For this review, use the dimensioned drawing (mm, ordinates from the lowest corner) and the shaded views. A direction names the side the tool comes from. Give positions to 0.01 mm unless a question says otherwise; leave off trailing zeros. Order: outer loops, then holes, each group sorted by start corner. A loop starts at its lowest first (then second) coordinate and runs counter-clockwise, first axis right, second up. Notation, with made-up numbers: (45, 1.25) -> (82, 1.25) arc R25 cw to (82, 38.25) -> close; hole circle Ø2 at (55, -20.75). An arc over 180 degrees is marked (long way). One line per item, written item: value. Start each with the question number.
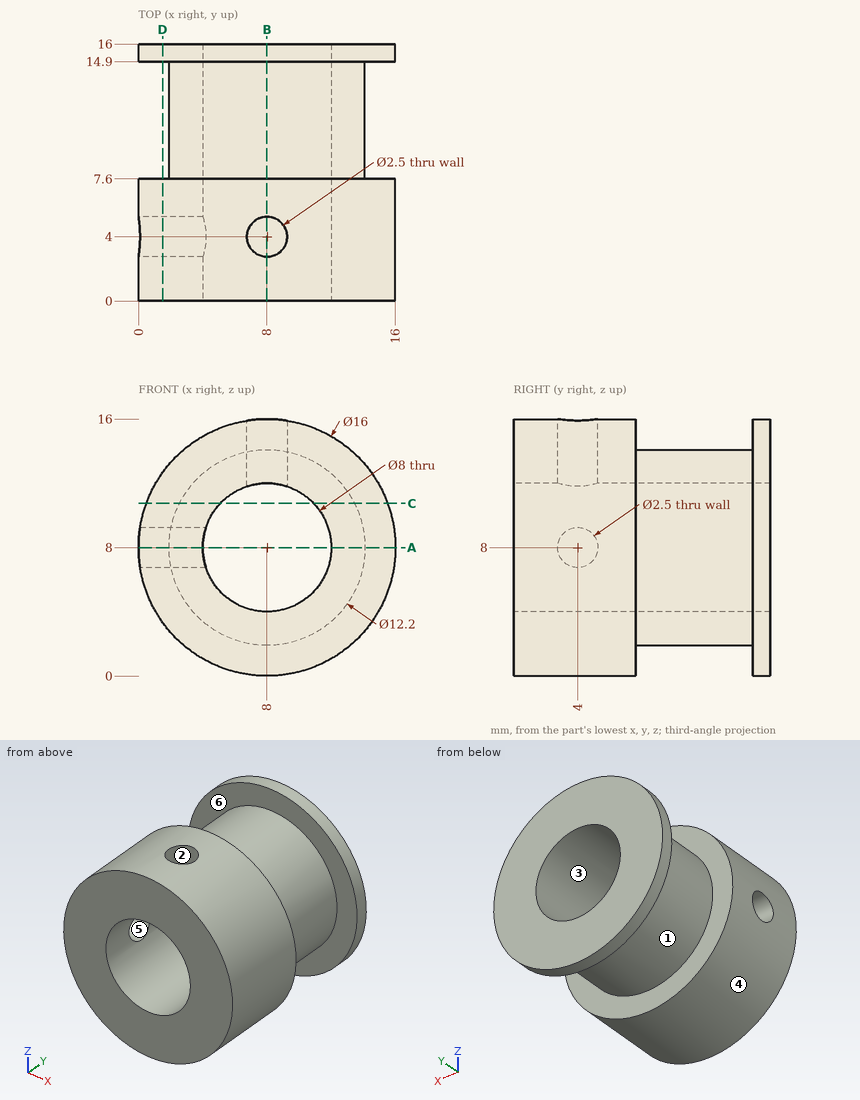
Q1. Take a section at C-C (z = 10.75). State the section outline as (x, y) points.
Q2. Take a section at B-B (x = 8). State the section outline as (y, z) points.
Q3. Take a section at D-D (x = 1.5). State the section outline as (y, z) points, and give its area (3 significant figures).
Q4. Take a section at A-A (z = 8). State the section outline as (x, y) points.
Q5. For the marked faces 4, 5 and 6, list the 3-axis set-ups (+Z, -Z, +X, -X, +Y, -Y) from which the entire face can be reached by the end or side of a thin tool; tool diameter is ignored.
Q6. For line 1 along X through (y, z) = (11.75, 8); line 2 along Y through (x, z) = (4.75, 15); line 3 along Z through (x, y) = (11, 10.5), list the stretches that pass through material, from the lowest coordinate up.
Q7. For pin 1 Ø6 at (y, z) = (7, 6.5) entering from +X; pin 2 Ø3 at (y, z) = (3.5, 10.5) entering from +X; pin 3 Ø4 at (x, y) = (11, 6) entering from -Z; pin 4 Ø3 at (x, y) = (13, 4) entering from +Z, all flat-tipped, find the tip position at first contact; note any pin that passes through.
Q8. Mouldability with a two-part tool opening along Z and no side actions: class the marked faces 1, 2 and 3 as pulls with the +Z half, pulls with the -Z half, needs draft (parallel to the pull), parting line crosses it, or undercut.
Answers below:
1. outline: (0.49, 0) -> (5.1, 0) -> (5.1, 16) -> (0.49, 16) -> (0.49, 14.9) -> (2.56, 14.9) -> (2.56, 7.6) -> (0.49, 7.6) -> close; (10.9, 0) -> (15.51, 0) -> (15.51, 7.6) -> (13.44, 7.6) -> (13.44, 14.9) -> (15.51, 14.9) -> (15.51, 16) -> (10.9, 16) -> close
2. outline: (0, 0) -> (7.6, 0) -> (7.6, 1.9) -> (14.9, 1.9) -> (14.9, 0) -> (16, 0) -> (16, 4) -> (0, 4) -> close; (0, 12) -> (2.75, 12) -> (2.75, 16) -> (0, 16) -> close; (5.25, 12) -> (16, 12) -> (16, 16) -> (14.9, 16) -> (14.9, 14.1) -> (7.6, 14.1) -> (7.6, 16) -> (5.25, 16) -> close
3. outline: (0, 3.34) -> (7.6, 3.34) -> (7.6, 12.66) -> (0, 12.66) -> close; (14.9, 3.34) -> (16, 3.34) -> (16, 12.66) -> (14.9, 12.66) -> close; hole circle Ø2.5 at (4, 8)
3. area: 76.2 mm²
4. outline: (0, 0) -> (4, 0) -> (4, 2.75) -> (0, 2.75) -> close; (0, 5.25) -> (4, 5.25) -> (4, 16) -> (0, 16) -> (0, 14.9) -> (1.9, 14.9) -> (1.9, 7.6) -> (0, 7.6) -> close; (12, 0) -> (16, 0) -> (16, 7.6) -> (14.1, 7.6) -> (14.1, 14.9) -> (16, 14.9) -> (16, 16) -> (12, 16) -> close
5. face 4: +Y, -Y
5. face 5: -X
5. face 6: none
6. line 1: x = 1.9 to 4, 12 to 14.1
6. line 2: y = 0 to 7.6, 14.9 to 16
6. line 3: z = 2.69 to 5.35, 10.65 to 13.31
7. pin 1: stops at x = 16
7. pin 2: stops at x = 15.94
7. pin 3: stops at z = 0.06
7. pin 4: stops at z = 15.19
8. face 1: parting line crosses it
8. face 2: needs draft
8. face 3: undercut
